Here's how the part is built. I have some questions about the finished solid (model axes, mm). Face numbers are marked on the shaded views. A direction names the side the tool comes from. Give positions to 0.01 mm unless a question says otherwise; leave off trailing zeros. Loops run counter-clockwise (first coordinate to the right, second up) from the corner with the lowest first, then second, coordinate; pieces in that order, holes last. Notation, with made-up numbers: (-15, -37.75) - (30, -37.75) arc R24 ccw to (30, -2.75) - close; hole circle Ø4 at (-22.75, 39). An arc over 180 degrees is marked (long way). Use one line per item in the form item = value.
from build123d import *

# Parameters (mm, degrees)
SKETCH2_R               = 45.4279
BOSS_EXTRUDE1_DEPTH     = 12.7
SKETCH3_R               = 12.7
BOSS_EXTRUDE2_DEPTH     = 8.89
SKETCH4_R               = 3.175
SKETCH4_R_2             = 1.1303
CUT_EXTRUDE1_DEPTH      = 22.59
SKETCH5_R               = 0.79375
CUT_EXTRUDE2_DEPTH      = 46.4279
CUT_EXTRUDE2_DEPTH_BACK = 46.4279
SKETCH6_R               = 1.1303
CUT_EXTRUDE3_DEPTH      = 13.7000001


with BuildPart() as part:
    # Sketch2 → Boss-Extrude1 (new body)
    with BuildSketch(Plane.XY):
        Circle(SKETCH2_R)
    extrude(amount=BOSS_EXTRUDE1_DEPTH)

    # Sketch3 → Boss-Extrude2 (add)
    with BuildSketch(Plane.XY.offset(12.7)):
        Circle(SKETCH3_R)
    extrude(amount=BOSS_EXTRUDE2_DEPTH)

    # Sketch4 → Cut-Extrude1 (cut, through all)
    with BuildSketch(Plane.XY.offset(21.59)):
        Circle(SKETCH4_R)
        with Locations((-7.9375, 0)):
            Circle(SKETCH4_R_2)
        with Locations((7.9375, 0)):
            Circle(SKETCH4_R_2)
    extrude(amount=-CUT_EXTRUDE1_DEPTH, mode=Mode.SUBTRACT)

    # Sketch5 → Cut-Extrude2 (cut, two sides)
    with BuildSketch(Plane(origin=(0, 0, 0), x_dir=(1, 0, 0), z_dir=(0, 1, 0))) as cut_extrude2_sk:
        with Locations((0, -17.145)):
            Circle(SKETCH5_R)
    extrude(amount=CUT_EXTRUDE2_DEPTH, mode=Mode.SUBTRACT)
    extrude(cut_extrude2_sk.sketch, amount=-CUT_EXTRUDE2_DEPTH_BACK, mode=Mode.SUBTRACT)

    # Sketch6 → Cut-Extrude3 (cut, through all)
    with BuildSketch(Plane.XY.offset(12.7)):
        with Locations((0, 25.4)):
            Circle(SKETCH6_R)
        with Locations((0, -25.4)):
            Circle(SKETCH6_R)
    extrude(amount=-CUT_EXTRUDE3_DEPTH, mode=Mode.SUBTRACT)


solid = part.part
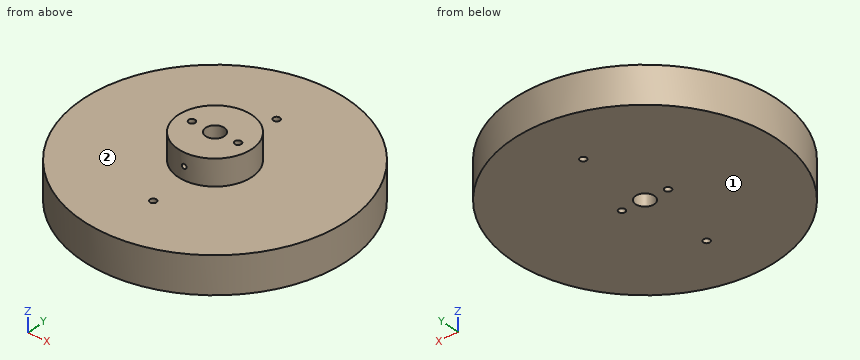
(1) If we section it at D-D (y = -10): List the corners of the cut face in (x, z) for me (1 decimal).
Geometry says:
outline = (-44.3, 0) - (44.3, 0) - (44.3, 12.7) - (7.8, 12.7) - (7.8, 21.6) - (-7.8, 21.6) - (-7.8, 12.7) - (-44.3, 12.7) - close; hole circle Ø1.6 at (0, 17.1)
(2) If I drill on probe 1 along Y at (x, z) = (0, 9.5) (3 decimals); probe 2 along Z at (x, y) = (0, -6); probe 3 along Y at (x, z) = (0, 16) (3 decimals), over which ranges is the centre line in solid material (lowest first)?
Geometry says:
probe_1 = -45.428 to -26.53, -24.27 to -3.175, 3.175 to 24.27, 26.53 to 45.428
probe_2 = 0 to 16.35, 17.94 to 21.59
probe_3 = -12.7 to -3.175, 3.175 to 12.7
(3) For the marked faces 1 and 2, which set-ups out of +Z, -Z, +X, -X, +Y, -Y let a thin tool reach every point of the face, with its end or its side?
Geometry says:
face_1 = -Z, +X, -X, +Y, -Y
face_2 = +Z
(4) If we section it at A-A (y = 0): List the corners of the cut face in (x, z) for me (3 decimals), plus the area to 3 significant figures.
Geometry says:
outline = (-45.428, 0) - (-9.068, 0) - (-9.068, 21.59) - (-12.7, 21.59) - (-12.7, 12.7) - (-45.428, 12.7) - close; (-6.807, 0) - (-3.175, 0) - (-3.175, 21.59) - (-6.807, 21.59) - close; (3.175, 0) - (6.807, 0) - (6.807, 21.59) - (3.175, 21.59) - close; (9.068, 0) - (45.428, 0) - (45.428, 12.7) - (12.7, 12.7) - (12.7, 21.59) - (9.068, 21.59) - close
area = 1,140 mm²
(5) For P1, Ø4, axis at x = 19.5, y = 30.5, coming from the +Z side; P2, Ø6, axis at x = 19, z = 3, coming from the +Y side; P3, Ø6, axis at x = -15, z = 2.5, coming from the -Y side, each with a flat end and sliding along its axis, tell me the tip position at first contact or that it passes through.
Geometry says:
P1 = 12.7
P2 = 42.52
P3 = -43.81
(6) If we section it at C-C (x = 5): List the corners of the cut face in (y, z) for me, plus the area to 3 significant figures.
Geometry says:
outline = (-45.15, 0) - (45.15, 0) - (45.15, 12.7) - (11.67, 12.7) - (11.67, 21.59) - (-11.67, 21.59) - (-11.67, 12.7) - (-45.15, 12.7) - close
area = 1,350 mm²
(7) If we section it at B-B (y = 25.4): List the corners of the cut face in (x, z) for me.
Geometry says:
outline = (-37.66, 0) - (-1.13, 0) - (-1.13, 12.7) - (-37.66, 12.7) - close; (1.13, 0) - (37.66, 0) - (37.66, 12.7) - (1.13, 12.7) - close
